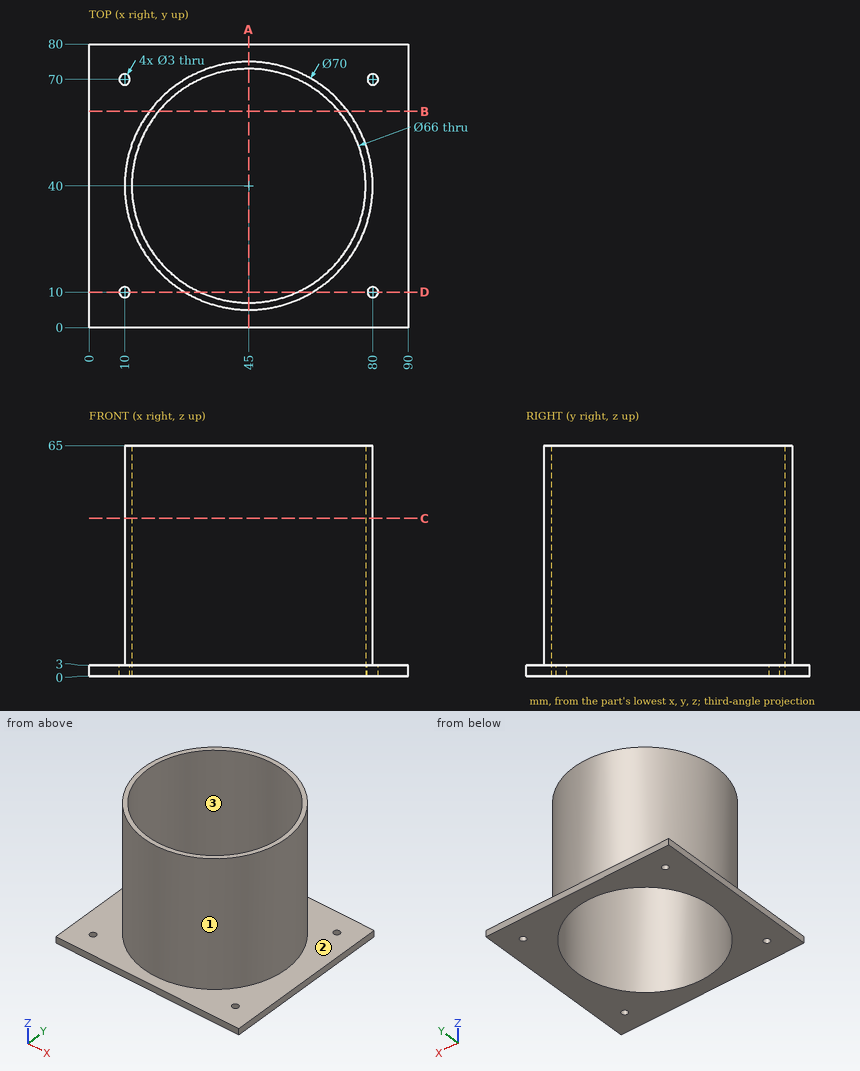
Geometry check sheet. Reference: drawing and pictorial views, mm from the part's lowest x, y, z. Give positions to 0.01 mm unless a question says otherwise; leave off trailing zeros. Order: outer loops, then holes, each group sorted by start corner. A loop starts at its lowest first (then second) coordinate and runs counter-clockwise, first axis right, second up. Notation, with made-up numbers: M -17,42.25 L 42,42.25 A17 cw 42,69.25 Z; hole C 71.5,7 d5. An arc over 180 degrees is marked long. Return JSON: item names as keys, results as strings. Group by question number.
1) Scan lines: line 1 (Y direction, x = 80, z = 1); line 2 (X direction, y = 10, z = 1.15); line 3 (Y direction, x = 45, z = 9). Record each from-to range of solid material in increasing order.
2) Section check C-C on z = 44.5. Record the cut outline in (x, y), and give its area (3 significant figures).
3) Section check D-D on y = 10. Record the cut outline in (x, z).
4) Section check B-B on y = 61. Record the cut outline in (x, z).
5) Section check A-A on x = 45. Record the cut outline in (y, z).
6) Go/stop test with flat-tipped pins: pin 1 Ø5 at (x, y) = (39, 68) entering from -Z; pin 2 Ø10 at (y, z) = (56, 11) entering from +X; pin 3 Ø1 at (x, z) = (43, 11.5) entering from -Y; pin 4 Ø10 at (x, z) = (33.5, 19.5) entering from +Y. Record where each tip stops, or that it passes through.
7) Mould release check, pull along Y, two halves, no side actions. Record for the marked faces 1, 2 and 3: pulls with the +Y half, pulls with the -Y half, needs draft (parallel to the pull), parting line crosses it, or undercut.
Answer block:
{
 "1": {"line 1": "y = 0 to 8.5, 11.5 to 68.5, 71.5 to 80", "line 2": "x = 0 to 8.5, 11.5 to 31.25, 58.75 to 78.5, 81.5 to 90", "line 3": "y = 5 to 7, 73 to 75"},
 "2": {"outline": "C 45,40 d70; hole C 45,40 d66", "area": "427 mm^2"},
 "3": {"outline": "M 0,0 L 8.5,0 L 8.5,3 L 0,3 Z; M 11.5,0 L 31.25,0 L 31.25,65 L 26.97,65 L 26.97,3 L 11.5,3 Z; M 58.75,0 L 78.5,0 L 78.5,3 L 63.03,3 L 63.03,65 L 58.75,65 Z; M 81.5,0 L 90,0 L 90,3 L 81.5,3 Z"},
 "4": {"outline": "M 0,0 L 19.54,0 L 19.54,65 L 17,65 L 17,3 L 0,3 Z; M 70.46,0 L 90,0 L 90,3 L 73,3 L 73,65 L 70.46,65 Z"},
 "5": {"outline": "M 0,0 L 7,0 L 7,65 L 5,65 L 5,3 L 0,3 Z; M 73,0 L 80,0 L 80,3 L 75,3 L 75,65 L 73,65 Z"},
 "6": {"pin 1": "passes through", "pin 2": "stops at x = 78.23", "pin 3": "stops at y = 5.03", "pin 4": "stops at y = 74.39"},
 "7": {"face 1": "parting line crosses it", "face 2": "needs draft", "face 3": "undercut"}
}
